Model file for the job. Use its own axes, mm. A direction names the side the tool comes from. Give positions to 0.01 mm unless a question says otherwise; leave off trailing zeros. Loops run counter-clockwise (first coordinate to the right, second up) from the corner with the lowest first, then second, coordinate; pieces in that order, holes last. Notation, with made-up numbers: (-4.5, 1) - (49.5, 1) arc R29 cw to (49.5, 36) - close; hole circle Ø11 at (-31.5, 6.25). An arc over 180 degrees is marked (long way). Use a Markdown table: item, result.
Autodesk Inventor part; units mm, degrees
ref_plane "YZ Plane" through (0, 0, 0) normal (1, 0, 0) x (0, 1, 0)
ref_plane "XZ Plane" through (0, 0, 0) normal (0, 1, 0) x (-1, 0, 0)
ref_plane "XY Plane" through (0, 0, 0) normal (0, 0, 1) x (1, 0, 0)
sketch "Sketch1" plane through (0, 0, 0) normal (0, 1, 0) x (-1, 0, 0)
  circle A0 centre (0, 0) radius 8.5
  circle A1 centre (5.1962, -3) radius 1.5
  circle A2 centre (5.1962, -3) radius 1.5
  circle A3 centre (-5.1962, -3) radius 1.5
  circle A4 centre (-5.1962, -3) radius 1.5
  circle A5 centre (0, 6) radius 1.5
  circle A6 centre (0, 6) radius 1.5
  point P0 (0, 0)
extrude "Extrusion1" add sketch "Sketch1" along normal blind 10
sketch "Sketch2" plane through (0, 10, 0) normal (0, 1, 0) x (1, 0, 0)
  circle A0 centre (0, 0) radius 2.5
  dimension "d3" = 5
extrude "Extrusion2" add sketch "Sketch2" along normal blind 30
thread "Thread1"
properties part number "Motor top"
(1) Slice it at A-A, the plane x = 0. Write the cut outline in (y, z), plus the area to 3 significant figures.
Computed:
| item | result |
|---|---|
| outline | (0, -8.5) - (10, -8.5) - (10, -2.5) - (40, -2.5) - (40, 2.5) - (10, 2.5) - (10, 4.5) - (0, 4.5) - close; (0, 7.5) - (10, 7.5) - (10, 8.5) - (0, 8.5) - close |
| area | 290 mm² |
(2) Slice it at C-C, the plane z = 6. Write the cut outline in (x, y), plus the area to 3 significant figures.
Computed:
| item | result |
|---|---|
| outline | (-6.02, 0) - (-1.5, 0) - (-1.5, 10) - (-6.02, 10) - close; (1.5, 0) - (6.02, 0) - (6.02, 10) - (1.5, 10) - close |
| area | 90.4 mm² |
(3) Pin check, flat tips, straight feed: P1, Ø8.5, axis at x = -2.5, z = 1.5, coming from the +Y side; P2, Ø1.5, axis at x = -2.5, z = 5, coming from the +Y side; P3, Ø4, axis at y = 26, z = -3.5, coming from the +X side; P4, Ø8, axis at y = 34, z = -4, coming from the +X side. Stop position of each tip, or through.
Computed:
| item | result |
|---|---|
| P1 | y = 40 |
| P2 | y = 10 |
| P3 | x = 2 |
| P4 | x = 2.5 |
(4) Drill centre lines: probe 1 along Z at (x, y) = (0, 5.5); probe 2 along Y at (x, z) = (4.75, 6); probe 3 along Z at (x, y) = (1, 25). Where is each one in solid material? Low to high. Write a range as [from, to].
Computed:
| item | result |
|---|---|
| probe 1 | [-8.5, 4.5], [7.5, 8.5] |
| probe 2 | [0, 10] |
| probe 3 | [-2.29, 2.29] |
(5) Slice it at D-D, the plane x = 4.75. Write the cut outline in (y, z).
Computed:
| item | result |
|---|---|
| outline | (0, -7.05) - (10, -7.05) - (10, -4.43) - (0, -4.43) - close; (0, -1.57) - (10, -1.57) - (10, 7.05) - (0, 7.05) - close |
(6) Mould opens along X. For faces 3 (the cylindrical face through (3.81, 4.93, -2.43)), 4 (the flat face through (0, 0, 0)), 5 (the cylindrical face through (-0.54, 24.79, -2.44)) say: pulls with the +X half, pulls with the -X half, needs draft (parallel to the pull), parting line crosses it, or undercut.
Computed:
| item | result |
|---|---|
| face 3 | undercut |
| face 4 | needs draft |
| face 5 | parting line crosses it |
(7) Slice it at B-B, the plane z = 0. Write the cut outline in (x, y), plus the area to 3 significant figures.
Computed:
| item | result |
|---|---|
| outline | (-8.5, 0) - (8.5, 0) - (8.5, 10) - (2.5, 10) - (2.5, 40) - (-2.5, 40) - (-2.5, 10) - (-8.5, 10) - close |
| area | 320 mm² |
(8) 3-axis set-ups, long thin cutter, end or side, ignore diameter. For faces 1 (the flat face through (-2, 10, -2)), 2 (the cylindrical face through (0.325, 4.93, 7.464)): which of +Z, -Z, +X, -X, +Y, -Y reach the whole face in a straight line?
Computed:
| item | result |
|---|---|
| face 1 | +Y |
| face 2 | +Y, -Y |
